Design review of the part shown in the three views and the two pictorial views. Dimensions are in mm from the part's minimum x, y and z. Give positions to 0.01 mm unless a question says otherwise; leave off trailing zeros. Write each loop counter-clockwise with the first axis right and the second up, starting at its lowest first coordinate (ties: lowest second). Pieces come first, ordered by that corner, then holes.
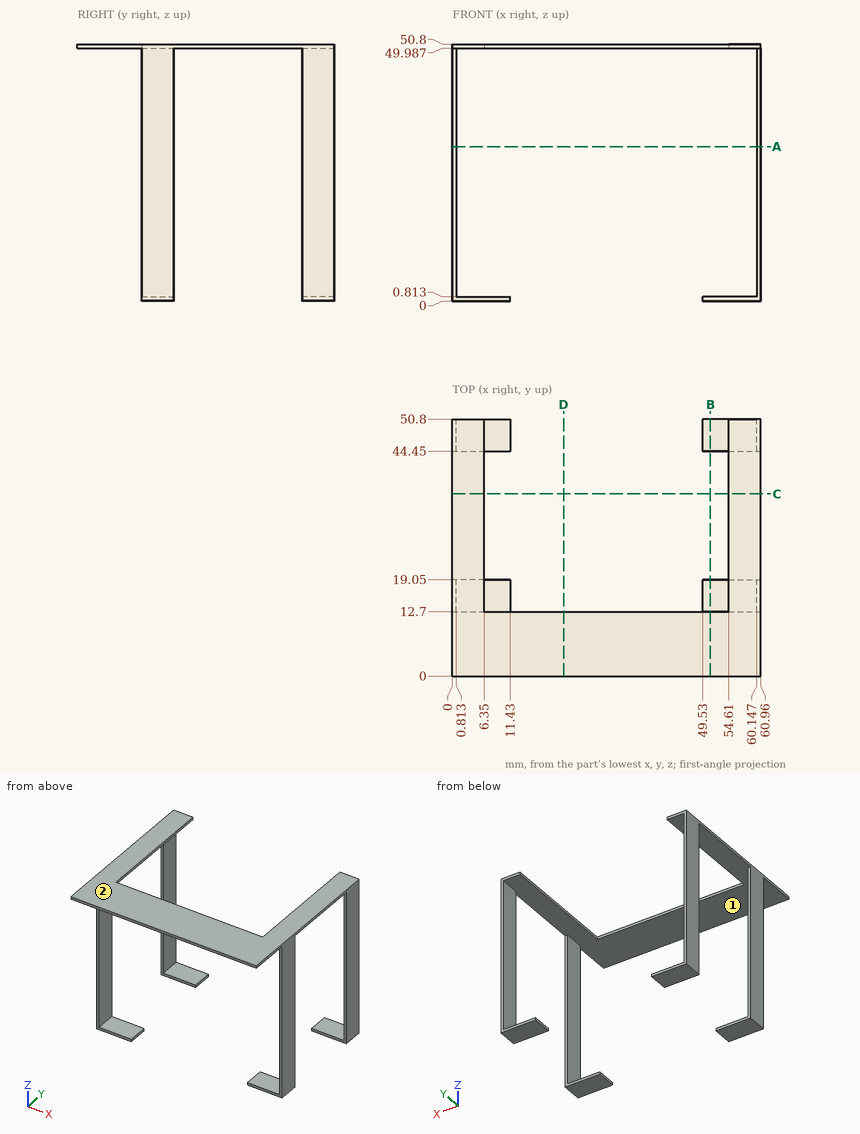
(1) Mouldability with a two-part tool opening along Z and no side actions: class the marked faces 1 and 2 as pulls with the +Z half, pulls with the -Z half, needs draft (parallel to the pull), parting line crosses it, or undercut.
Resolved:
face 1: undercut
face 2: pulls with the +Z half
(2) Consider section D-D, the plane x = 22. Give the boundary of the cut face in (y, z).
Resolved:
outline: (0, 49.99) - (12.7, 49.99) - (12.7, 50.8) - (0, 50.8) - close
(3) Consider section B-B, the plane x = 51. Give the boundary of the cut face in (y, z).
Resolved:
outline: (0, 49.99) - (12.7, 49.99) - (12.7, 50.8) - (0, 50.8) - close; (12.7, 0) - (19.05, 0) - (19.05, 0.81) - (12.7, 0.81) - close; (44.45, 0) - (50.8, 0) - (50.8, 0.81) - (44.45, 0.81) - close
(4) To check wall thickness, follow L1, parallel to X at y = 16, z = 9; L2, parallel to Z at x = 38.5, y = 6. State the ranges of each line that lie inside material, in increasing order.
Resolved:
L1: x = 0 to 0.81, 60.15 to 60.96
L2: z = 49.99 to 50.8
(5) Clearance check with flat-ended pins moving along their axes: P1, Ø3, axis at x = 7.5, y = 46, coming from the +Z side; P2, Ø12.5, axis at x = 54.5, z = 21, coming from the -Y side; P3, Ø4, axis at x = 52.5, y = 16.5, coming from the +Z side. State where each tip first meets the part, or that it passes through.
Resolved:
P1: stops at z = 50.8
P2: stops at y = 12.7
P3: stops at z = 0.81
(6) Consider section A-A, the plane z = 30.5. Give the boundary of the cut face in (x, y).
Resolved:
outline: (0, 12.7) - (0.81, 12.7) - (0.81, 19.05) - (0, 19.05) - close; (0, 44.45) - (0.81, 44.45) - (0.81, 50.8) - (0, 50.8) - close; (60.15, 12.7) - (60.96, 12.7) - (60.96, 19.05) - (60.15, 19.05) - close; (60.15, 44.45) - (60.96, 44.45) - (60.96, 50.8) - (60.15, 50.8) - close
(7) Consider section C-C, the plane y = 36. Give the boundary of the cut face in (x, z).
Resolved:
outline: (0, 49.99) - (6.35, 49.99) - (6.35, 50.8) - (0, 50.8) - close; (54.61, 49.99) - (60.96, 49.99) - (60.96, 50.8) - (54.61, 50.8) - close
